from build123d import *

# Parameters (mm, degrees)
SKETCH_1_W          = 100
SKETCH_1_H          = 100
SKETCH_1_R          = 1.5
EXTRUDE_1_DEPTH     = 3
SKETCH_4_W          = 100
SKETCH_4_H          = 100
EXTRUDE_4_DEPTH     = 23
SKETCH_5_R          = 4
SKETCH_5_R_2        = 1.5
EXTRUDE_5_DEPTH     = 13
FILLET_2_R          = 2
FILLET_3_R          = 8
SKETCH_7_R          = 1.5
EXTRUDE_6_DEPTH     = 23
SKETCH_8_R          = 1.75
SKETCH_8_R_2        = 2
CUT_EXTRUDE_2_DEPTH = 3
SKETCH_9_R          = 3.25
CUT_EXTRUDE_3_DEPTH = 2.5
CUT_EXTRUDE_4_DEPTH = 2.5


with BuildPart() as part:
    # Эскиз1 → Бобышка-Вытянуть1 (new body)
    with BuildSketch(Plane(origin=(0, 0, 0), x_dir=(1, 0, 0), z_dir=(0, 1, 0))):
        with Locations((50, 50)):
            Rectangle(SKETCH_1_W, SKETCH_1_H)
        with Locations(Location((14.7, 81, 0), (0, 0, 270))):
            Circle(SKETCH_1_R, mode=Mode.SUBTRACT)
        with Locations(Location((71.7, 75, 0), (0, 0, 270))):
            Circle(SKETCH_1_R, mode=Mode.SUBTRACT)
        with Locations(Location((71.7, 25, 0), (0, 0, 90))):
            Circle(SKETCH_1_R, mode=Mode.SUBTRACT)
        with Locations(Location((14.7, 19, 0), (0, 0, 90))):
            Circle(SKETCH_1_R, mode=Mode.SUBTRACT)
        with Locations(Location((7, 93, 0), (0, 0, 270))):
            Circle(SKETCH_1_R, mode=Mode.SUBTRACT)
        with Locations(Location((93, 93, 0), (0, 0, 90))):
            Circle(SKETCH_1_R, mode=Mode.SUBTRACT)
        with Locations(Location((93, 7, 0), (0, 0, 270))):
            Circle(SKETCH_1_R, mode=Mode.SUBTRACT)
        with Locations(Location((7, 7, 0), (0, 0, 90))):
            Circle(SKETCH_1_R, mode=Mode.SUBTRACT)
    extrude(amount=EXTRUDE_1_DEPTH)

    # Эскиз4 → Бобышка-Вытянуть4 (add)
    with BuildSketch(Plane(origin=(0, 3, 0), x_dir=(1, 0, 0), z_dir=(0, 1, 0))):
        with Locations((50, 50)):
            Rectangle(SKETCH_4_W, SKETCH_4_H)
        with BuildLine():
            Line((97, 97), (3, 97))
            Line((3, 97), (3, 65.304901176))
            ThreePointArc((3, 65.304901176), (2.879271228, 63.755707837), (2.52, 62.243920941))
            ThreePointArc((2.52, 62.243920941), (0.6, 50), (2.52, 37.756079059))
            ThreePointArc((2.52, 37.756079059), (2.879271228, 36.244292163), (3, 34.695098824))
            Line((3, 34.695098824), (3, 3))
            Line((3, 3), (97, 3))
            Line((97, 3), (97, 37.262653338))
            ThreePointArc((97, 37.262653338), (97.172923702, 39.114293537), (97.685714286, 40.901895241))
            ThreePointArc((97.685714286, 40.901895241), (99.4, 50), (97.685714286, 59.098104759))
            ThreePointArc((97.685714286, 59.098104759), (97.172923702, 60.885706463), (97, 62.737346662))
            Line((97, 62.737346662), (97, 97))
        make_face(mode=Mode.SUBTRACT)
    extrude(amount=EXTRUDE_4_DEPTH)

    # Эскиз5 → Бобышка-Вытянуть5 (add)
    # profile 1 of 4: a face of its own
    with BuildSketch(Plane(origin=(0, 3, 0), x_dir=(1, 0, 0), z_dir=(0, 1, 0))):
        with Locations(Location((14.7, 81, 0), (0, 0, 90))):
            Circle(SKETCH_5_R)
        with Locations(Location((14.7, 81, 0), (0, 0, 270))):
            Circle(SKETCH_5_R_2, mode=Mode.SUBTRACT)
    # profile 2 of 4: a face of its own
    with BuildSketch(Plane(origin=(0, 3, 0), x_dir=(1, 0, 0), z_dir=(0, 1, 0))):
        with Locations(Location((71.7, 75, 0), (0, 0, 90))):
            Circle(SKETCH_5_R)
        with Locations(Location((71.7, 75, 0), (0, 0, 270))):
            Circle(SKETCH_5_R_2, mode=Mode.SUBTRACT)
    # profile 3 of 4: a face of its own
    with BuildSketch(Plane(origin=(0, 3, 0), x_dir=(1, 0, 0), z_dir=(0, 1, 0))):
        with Locations(Location((71.7, 25, 0), (0, 0, 90))):
            Circle(SKETCH_5_R)
        with Locations(Location((71.7, 25, 0), (0, 0, 90))):
            Circle(SKETCH_5_R_2, mode=Mode.SUBTRACT)
    # profile 4 of 4: a face of its own
    with BuildSketch(Plane(origin=(0, 3, 0), x_dir=(1, 0, 0), z_dir=(0, 1, 0))):
        with Locations(Location((14.7, 19, 0), (0, 0, 90))):
            Circle(SKETCH_5_R)
        with Locations(Location((14.7, 19, 0), (0, 0, 90))):
            Circle(SKETCH_5_R_2, mode=Mode.SUBTRACT)
    extrude(amount=EXTRUDE_5_DEPTH)

    # Скругление2
    fillet_2_edges = [part.edges().sort_by_distance(p)[0] for p in [
        (71.7, 3, -21),
        (14.7, 3, -15),
        (14.7, 3, -77),
        (71.7, 3, -71),
    ]]
    fillet(fillet_2_edges, radius=FILLET_2_R)

    # Скругление3
    fillet_3_edges = [part.edges().sort_by_distance(p)[0] for p in [
        (0, 13, -100),
        (100, 13, -100),
        (100, 13, 0),
        (0, 13, 0),
    ]]
    fillet(fillet_3_edges, radius=FILLET_3_R)

    # Эскиз7 → Бобышка-Вытянуть6 (add)
    # profile 1 of 4: a face of its own
    with BuildSketch(Plane(origin=(0, 3, 0), x_dir=(1, 0, 0), z_dir=(0, 1, 0))):
        with BuildLine():
            Line((3, 89), (3, 97))
            Line((3, 97), (11, 97))
            Line((11, 97), (11, 93))
            ThreePointArc((11, 93), (9.828427125, 90.171572875), (7, 89))
            Line((7, 89), (3, 89))
        make_face()
        with Locations(Location((7, 93, 0), (0, 0, 270))):
            Circle(SKETCH_7_R, mode=Mode.SUBTRACT)
    # profile 2 of 4: a face of its own
    with BuildSketch(Plane(origin=(0, 3, 0), x_dir=(1, 0, 0), z_dir=(0, 1, 0))):
        with BuildLine():
            Line((89, 93), (89, 97))
            Line((89, 97), (97, 97))
            Line((97, 97), (97, 89))
            Line((97, 89), (93, 89))
            ThreePointArc((93, 89), (90.171572875, 90.171572875), (89, 93))
        make_face()
        with Locations(Location((93, 93, 0), (0, 0, 90))):
            Circle(SKETCH_7_R, mode=Mode.SUBTRACT)
    # profile 3 of 4: a face of its own
    with BuildSketch(Plane(origin=(0, 3, 0), x_dir=(1, 0, 0), z_dir=(0, 1, 0))):
        with BuildLine():
            Line((97, 11), (97, 3))
            Line((97, 3), (89, 3))
            Line((89, 3), (89, 7))
            ThreePointArc((89, 7), (90.171572875, 9.828427125), (93, 11))
            Line((93, 11), (97, 11))
        make_face()
        with Locations(Location((93, 7, 0), (0, 0, 270))):
            Circle(SKETCH_7_R, mode=Mode.SUBTRACT)
    # profile 4 of 4: a face of its own
    with BuildSketch(Plane(origin=(0, 3, 0), x_dir=(1, 0, 0), z_dir=(0, 1, 0))):
        with BuildLine():
            Line((11, 7), (11, 3))
            Line((11, 3), (3, 3))
            Line((3, 3), (3, 11))
            Line((3, 11), (7, 11))
            ThreePointArc((7, 11), (9.828427125, 9.828427125), (11, 7))
        make_face()
        with Locations(Location((7, 7, 0), (0, 0, 90))):
            Circle(SKETCH_7_R, mode=Mode.SUBTRACT)
    extrude(amount=EXTRUDE_6_DEPTH)

    # Эскиз8 → Вырез-Вытянуть2 (cut)
    with BuildSketch(Plane(origin=(0, 3, 0), x_dir=(1, 0, 0), z_dir=(0, 1, 0))):
        with Locations(Location((20, 90, 0), (0, 0, 270))):
            Circle(SKETCH_8_R)
        with Locations(Location((80, 90, 0), (0, 0, 90))):
            Circle(SKETCH_8_R)
        with Locations(Location((80, 10, 0), (0, 0, 270))):
            Circle(SKETCH_8_R)
        with Locations(Location((20, 10, 0), (0, 0, 90))):
            Circle(SKETCH_8_R)
        with Locations(Location((22.592071992, 61.508405751, 0), (0, 0, 270))):
            Circle(SKETCH_8_R_2)
        with Locations(Location((12.592071992, 61.508405751, 0), (0, 0, 270))):
            Circle(SKETCH_8_R_2)
        with BuildLine():
            Line((12.592071992, 57.5), (87.592071992, 57.5))
            ThreePointArc((87.592071992, 57.5), (95.092071992, 50), (87.592071992, 42.5))
            Line((87.592071992, 42.5), (12.592071992, 42.5))
            ThreePointArc((12.592071992, 42.5), (5.092071992, 50), (12.592071992, 57.5))
        make_face()
    extrude(amount=-CUT_EXTRUDE_2_DEPTH, mode=Mode.SUBTRACT)

    # Эскиз9 → Вырез-Вытянуть3 (cut)
    with BuildSketch(Plane.XZ):
        with Locations(Location((7, -7, 0), (0, 0, 270))):
            Circle(SKETCH_9_R)
        with Locations(Location((93, -7, 0), (0, 0, 270))):
            Circle(SKETCH_9_R)
        with Locations(Location((93, -93, 0), (0, 0, 270))):
            Circle(SKETCH_9_R)
        with Locations(Location((7, -93, 0), (0, 0, 270))):
            Circle(SKETCH_9_R)
    extrude(amount=-CUT_EXTRUDE_3_DEPTH, mode=Mode.SUBTRACT)

    # Эскиз10 → Вырез-Вытянуть4 (cut)
    with BuildSketch(Plane(origin=(0, 26, 0), x_dir=(1, 0, 0), z_dir=(0, 1, 0))):
        Polygon((8.616580754, 90.2), (10.233161507, 93), (8.616580754, 95.8), (5.383419246, 95.8), (3.766838493, 93), (5.383419246, 90.2), align=None)
        Polygon((94.616580754, 90.2), (91.383419246, 90.2), (89.766838493, 93), (91.383419246, 95.8), (94.616580754, 95.8), (96.233161507, 93), align=None)
        Polygon((91.383419246, 9.8), (89.766838493, 7), (91.383419246, 4.2), (94.616580754, 4.2), (96.233161507, 7), (94.616580754, 9.8), align=None)
        Polygon((5.383419246, 9.8), (8.616580754, 9.8), (10.233161507, 7), (8.616580754, 4.2), (5.383419246, 4.2), (3.766838493, 7), align=None)
    extrude(amount=-CUT_EXTRUDE_4_DEPTH, mode=Mode.SUBTRACT)


solid = part.part
Verification items for the finished model (mm, model axes). A direction names the side the tool comes from. Coordinates: 2 decimals unless noted, no trailing zeros. Write each loop counter-clockwise with the first axis right and the second up, starting at its lowest first coordinate (ties: lowest second). Pieces come first, ordered by that corner, then holes. Notation, with made-up numbers: M -21,0 L 26,0 A24 cw 26,26 Z; hole C 32.5,22 d8. An arc over 180 degrees is marked long. Use CSV: the item, a comma, the result in double quotes.
Q1. Section check C-C, the plane x = 50. Enter the section's corners in (y, z).
Computed values:
outline,"M 0,-100 L 26,-100 L 26,-97 L 3,-97 L 3,-57.5 L 0,-57.5 Z; M 0,-42.5 L 3,-42.5 L 3,-3 L 26,-3 L 26,0 L 0,0 Z"
Q2. Go/stop test with flat-tipped pins: P1, Ø4, axis at x = 27, z = -22, coming from the +Y side; P2, Ø1.2, axis at x = 95.5, y = 9, coming from the +Z side; P3, Ø1.2, axis at x = 93, y = 24.5, coming from the +Z side. Record where each tip stops, or that it passes through.
Computed values:
P1,"y = 3"
P2,"z = -0.54"
P3,"z = -0.01"
Q3. Section check A-A, the plane x = 71.7. State how many separate pieces and enclosed holes the cut face has, and give its area (3 significant figures).
Computed values:
separate pieces,"4"
enclosed holes,"0"
area,"508 mm²"
Q4. Thickness scan on line 1 along Z through (x, y) = (71.7, 10.25); line 2 along Z through (x, y) = (66.5, 17.75); line 3 along Z through (x, y) = (11, 2.25). Record the ranges inside material, lowest first. Write a range as [from, to].
Computed values:
line 1,"[-100, -97], [-79, -76.5], [-73.5, -71], [-29, -26.5], [-23.5, -21], [-3, 0]"
line 2,"[-100, -97], [-3, 0]"
line 3,"[-100, -62.72], [-60.3, -57.33], [-42.67, 0]"
Q5. Mould release check, pull along X, two halves, no side actions. Record for faces 4 (the flat face through (49, 13, -100)), 5 (the flat face through (7, 25, -9.8)), 6 (the flat face through (100, 13, -49)): pulls with the +X half, pulls with the -X half, needs draft (parallel to the pull), parting line crosses it, or undercut.
Computed values:
face 4,"needs draft"
face 5,"undercut"
face 6,"pulls with the +X half"
Q6. Set-up check for faces 1 (the flat face through (51, 2, -42.5)), 2 (the flat face through (92.3, 2.5, -91.5)), 3 (the flat face through (11, 14, -95)): record each of +Z, -Z, +X, -X, +Y, -Y from which the full face is reachable in a straight line by a thin tool's end or side.
Computed values:
face 1,"+Y, -Y"
face 2,"-Y"
face 3,"+Y"
